Verification items for the finished model (mm, model axes). Coordinates: 2 decimals unless noted, no trailing zeros. Write each loop counter-clockwise with the first axis right and the second up, starting at its lowest first coordinate (ties: lowest second). Pieces come first, ordered by that corner, then holes. Notation, with made-up numbers: (83.25, 3.5) -> (128.25, 3.5) arc R10 ccw to (128.25, 8.5) -> close; hole circle Ø5 at (17.5, -5). An arc over 180 degrees is marked (long way). Answer in a Markdown table with one row per item.
```python
from build123d import *

# Parameters (mm, degrees)
BOSS_EXTRUDE1_DEPTH = 3.175
SKETCH2_R           = 2.54
CUT_EXTRUDE1_DEPTH  = 3.175


with BuildPart() as part:
    # Sketch1 → Boss-Extrude1 (new body)
    with BuildSketch(Plane(origin=(0, 0, 0), x_dir=(1, 0, 0), z_dir=(0, 1, 0))):
        Polygon((-38.1, -50.8), (12.7, -50.8), (12.7, 0), (12.7, 50.8), (-38.1, 50.8), align=None)
    extrude(amount=BOSS_EXTRUDE1_DEPTH)

    # Sketch2 → Cut-Extrude1 (cut)
    with BuildSketch(Plane(origin=(0, 3.175, 0), x_dir=(1, 0, 0), z_dir=(0, 1, 0))):
        with Locations(Location((-25.4, 38.1, 0), (0, 0, 270))):
            Circle(SKETCH2_R)
        with Locations(Location((-25.4, 12.7, 0), (0, 0, 270))):
            Circle(SKETCH2_R)
        with Locations(Location((-25.4, -12.7, 0), (0, 0, 270))):
            Circle(SKETCH2_R)
        with Locations(Location((-25.4, -38.1, 0), (0, 0, 270))):
            Circle(SKETCH2_R)
        with Locations(Location((0, 12.7, 0), (0, 0, 270))):
            Circle(SKETCH2_R)
        with Locations(Location((0, -12.7, 0), (0, 0, 270))):
            Circle(SKETCH2_R)
        with Locations(Location((0, -38.1, 0), (0, 0, 270))):
            Circle(SKETCH2_R)
        with Locations(Location((0, 38.1, 0), (0, 0, 270))):
            Circle(SKETCH2_R)
    extrude(amount=-CUT_EXTRUDE1_DEPTH, mode=Mode.SUBTRACT)


solid = part.part
```
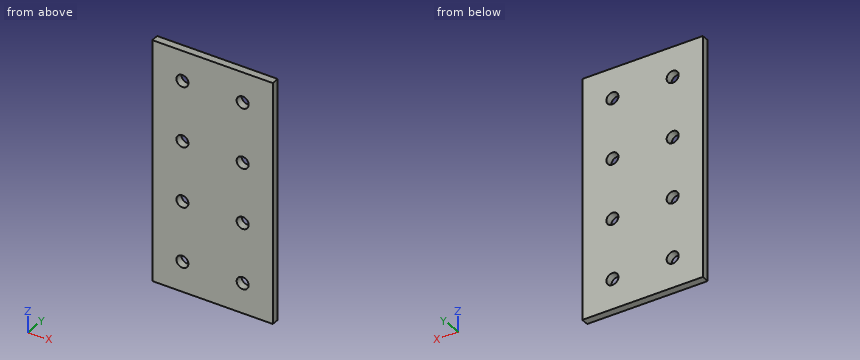
1. Sectioned sample at B-B, the plane x = 0. Record the cut outline in (y, z) (3 decimals).
Findings below:
| item | result |
|---|---|
| outline | (0, -50.8) -> (3.175, -50.8) -> (3.175, -40.64) -> (0, -40.64) -> close; (0, -35.56) -> (3.175, -35.56) -> (3.175, -15.24) -> (0, -15.24) -> close; (0, -10.16) -> (3.175, -10.16) -> (3.175, 10.16) -> (0, 10.16) -> close; (0, 15.24) -> (3.175, 15.24) -> (3.175, 35.56) -> (0, 35.56) -> close; (0, 40.64) -> (3.175, 40.64) -> (3.175, 50.8) -> (0, 50.8) -> close |
2. Sectioned sample at D-D, the plane z = 13.5. Record the cut outline in (x, y) (3 decimals), and give its area (3 significant figures).
Findings below:
| item | result |
|---|---|
| outline | (-38.1, 0) -> (-27.811, 0) -> (-27.811, 3.175) -> (-38.1, 3.175) -> close; (-22.989, 0) -> (-2.411, 0) -> (-2.411, 3.175) -> (-22.989, 3.175) -> close; (2.411, 0) -> (12.7, 0) -> (12.7, 3.175) -> (2.411, 3.175) -> close |
| area | 131 mm² |
3. Material ranges on probe 1 along X at (y, z) = (2.25, -38.1); probe 2 along Z at (x, y) = (-27.5, 2.7); probe 3 along X at (y, z) = (1.15, 14.5), recorded low to high. Write a range as from..to.
Findings below:
| item | result |
|---|---|
| probe 1 | x = -38.1..-27.94, -22.86..-2.54, 2.54..12.7 |
| probe 2 | z = -50.8..-39.53, -36.67..-14.13, -11.27..11.27, 14.13..36.67, 39.53..50.8 |
| probe 3 | x = -38.1..-27.19, -23.61..-1.79, 1.79..12.7 |
4. Sectioned sample at C-C, the plane y = 0.7. Count the separate pieces of the cut face and the enclosed holes in it, and give its area (3 significant figures).
Findings below:
| item | result |
|---|---|
| separate pieces | 1 |
| enclosed holes | 8 |
| area | 5,000 mm² |
5. Sectioned sample at A-A, the plane z = -38.1. Record the cut outline in (x, y) (3 decimals).
Findings below:
| item | result |
|---|---|
| outline | (-38.1, 0) -> (-27.94, 0) -> (-27.94, 3.175) -> (-38.1, 3.175) -> close; (-22.86, 0) -> (-2.54, 0) -> (-2.54, 3.175) -> (-22.86, 3.175) -> close; (2.54, 0) -> (12.7, 0) -> (12.7, 3.175) -> (2.54, 3.175) -> close |
6. Go/stop test with a flat-tipped pin: pin 1 (12 mm diameter, centred on x = -27.5, z = 17, fed in from -Y). Record where the tip stops, or that it passes through.
Findings below:
| item | result |
|---|---|
| pin 1 | stops at y = 0 |
